Autodesk Inventor part; units mm, degrees
ref_plane "YZ Plane" through (0, 0, 0) normal (1, 0, 0) x (0, 1, 0)
ref_plane "XZ Plane" through (0, 0, 0) normal (0, 1, 0) x (-1, 0, 0)
ref_plane "XY Plane" through (0, 0, 0) normal (0, 0, 1) x (1, 0, 0)
sketch "Sketch1" plane through (0, 0, 0) normal (0, 1, 0) x (-1, 0, 0)
  circle A0 centre (0, 0) radius 36
  line L0 (-22.225, 22.225) -> (22.225, 22.225)
  line L1 (22.225, 22.225) -> (22.225, -22.225)
  line L2 (22.225, -22.225) -> (-22.225, -22.225)
  line L3 (-22.225, -22.225) -> (-22.225, 22.225)
  line L4 (-22.225, 22.225) -> (22.225, -22.225) construction
  line L5 (22.225, 22.225) -> (-22.225, -22.225) construction
  circle A1 centre (0, 0) radius 32.5
  circle A2 centre (22.225, -22.225) radius 2.25
  circle A3 centre (22.225, 22.225) radius 2.25
  circle A4 centre (-22.225, 22.225) radius 2.25
  circle A5 centre (-22.225, -22.225) radius 2.25
  line L6 (-25.512, 25.3996) -> (-25.512, -25.3996)
  dimension "d0" = 72
  dimension "d1" = 44.45
  dimension "d2" = 44.45
  dimension "d3" = 65
  dimension "d4" = 4.5
  dimension "d5" = 4.5
  dimension "d6" = 4.5
  dimension "d7" = 4.5
  dimension "d9" = 25.512
  dimension "d10" = 3.287
extrude "Extrusion1" add sketch "Sketch1" along normal blind 10 contours A0 L6 A1 A5 A2 A3 A4 | A1 A4 L3 A5 L6 | A1 A3 L0 A4 | A4 L0 A3 L1 A2 L2 A5 L3 | A5 L2 A2 A1 | A1 A2 L1 A3
sketch "Sketch2" plane through (0, 10, 0) normal (0, 1, 0) x (1, 0, 0)
  circle A0 centre (0, 0) radius 2.5
  dimension "d13" = 5
extrude "Extrusion2" cut sketch "Sketch2" against normal blind 10
properties part number "Bottom Cap outlet"
Geometry: final body of the model. Coordinates: model frame, mm. Give positions to 0.01 mm unless a question says otherwise; leave off trailing zeros. Write each loop counter-clockwise with the first axis right and the second up, starting at its lowest first coordinate (ties: lowest second). Pieces come first, ordered by that corner, then holes.
1. Section query D-D, the plane x = -6.5. Return loops of the section in (y, z), then the cut area to 3 significant figures.
2. Line query: probe 1 along X at (y, z) = (6.5, 0); probe 2 along Z at (x, y) = (-21, 1.5); probe 3 along X at (y, z) = (9.5, 24). Output: solid intervals per line, ascending.
3. Draft query along Z for faces 1 (the flat face through (-5, 10, 1)), 2 (the cylindrical face through (-35.98, 4.93, 1.19)), 3 (the cylindrical face through (21.015, 4.93, 20.328)). Return one class per face: released by +Z, released by -Z, zero draft, split by the parting line, or undercut.
4. Pin query (flat end, axial travel): P1, Ø3.5, axis at x = -22.225, z = -22.225, coming from the -Y side; P2, Ø3, axis at x = -21.5, y = 3, coming from the -Z side; P3, Ø4, axis at x = 13.5, y = 3, coming from the -Z side; P4, Ø6, axis at x = 15.5, y = 3.5, coming from the -Z side. Return the tip coordinate at first contact, or that it passes through.
5. Section query C-C, the plane y = 6.5. Return loops of the section in (x, z) (3 decimals), then the cut area to 3 significant figures.
6. Section query B-B, the plane z = 0. Return loops of the section in (x, y), then the cut area to 3 significant figures.
7. Section query A-A, the plane x = 0. Return loops of the section in (y, z), then the cut area to 3 significant figures.
Computed:
1. outline: (0, -35.41) - (10, -35.41) - (10, 35.41) - (0, 35.41) - close
1. area: 708 mm2
2. probe 1: x = -36 to -2.5, 2.5 to 25.51
2. probe 2: z = -29.24 to -24.11, -20.34 to 20.34, 24.11 to 29.24
2. probe 3: x = -26.83 to -23.61, -20.84 to 20.84, 23.61 to 25.51
3. face 1: zero draft
3. face 2: split by the parting line
3. face 3: undercut
4. P1: passes through
4. P2: stops at z = -29.93
4. P3: stops at z = -34.11
4. P4: stops at z = -33.76
5. outline: (25.512, -25.4) - (25.512, 25.4) arc R36 ccw (long way) to start; hole circle Ø4.5 at (-22.225, -22.225); hole circle Ø4.5 at (-22.225, 22.225); hole circle Ø5 at (0, 0); hole circle Ø4.5 at (22.225, -22.225); hole circle Ø4.5 at (22.225, 22.225)
5. area: 3,620 mm2
6. outline: (-36, 0) - (-2.5, 0) - (-2.5, 10) - (-36, 10) - close; (2.5, 0) - (25.51, 0) - (25.51, 10) - (2.5, 10) - close
6. area: 565 mm2
7. outline: (0, -36) - (10, -36) - (10, -2.5) - (0, -2.5) - close; (0, 2.5) - (10, 2.5) - (10, 36) - (0, 36) - close
7. area: 670 mm2
